from build123d import *

# Parameters (mm, degrees)
BOSS_EXTRUDE2_DEPTH     = 50.8
SKETCH2_R               = 12.7
CUT_EXTRUDE1_DEPTH      = 3.175
SKETCH3_R               = 6.35
CUT_EXTRUDE2_DEPTH      = 118.131253835
CUT_EXTRUDE3_DEPTH      = 117.397422652
CUT_EXTRUDE3_DEPTH_BACK = 117.397422652
SKETCH5_R               = 3.175
CUT_EXTRUDE4_DEPTH      = 118.946015193


with BuildPart() as part:
    # Sketch1 → Boss-Extrude2 (new body)
    with BuildSketch(Plane.XY):
        with BuildLine():
            Line((29.919216233, -6.35), (24.593444248, -6.35))
            ThreePointArc((24.593444248, -6.35), (23.905382985, -8.584443158), (23.014781645, -10.746154003))
            ThreePointArc((23.014781645, -10.746154003), (25.826619655, -7.542321317), (29.919216233, -6.35))
        make_face()
        with BuildLine():
            ThreePointArc((23.01478179, 10.746153692), (23.905383043, 8.584442996), (24.593444248, 6.35))
            Line((24.593444248, 6.35), (29.919216228, 6.35))
            ThreePointArc((29.919216228, 6.35), (25.826619797, 7.542321227), (23.01478179, 10.746153692))
        make_face()
        with BuildLine():
            Line((29.919216228, 6.35), (24.593444248, 6.35))
            ThreePointArc((24.593444248, 6.35), (25.197554285, 3.200509029), (25.4, 0))
            ThreePointArc((25.4, 0), (25.197554285, -3.200509029), (24.593444248, -6.35))
            Line((24.593444248, -6.35), (29.919216233, -6.35))
            Line((29.919216233, -6.35), (101.6, -6.35))
            Line((101.6, -6.35), (101.6, 6.35))
            Line((101.6, 6.35), (29.919216228, 6.35))
        make_face()
        with BuildLine():
            Line((24.593444248, -6.35), (0, -6.35))
            Line((0, -6.35), (0, -25.4))
            ThreePointArc((0, -25.4), (13.641988278, -21.425595811), (23.014781645, -10.746154003))
            ThreePointArc((23.014781645, -10.746154003), (23.905382985, -8.584443158), (24.593444248, -6.35))
        make_face()
        with BuildLine():
            Line((24.593444248, 6.35), (0, 6.35))
            Line((0, 6.35), (0, -6.35))
            Line((0, -6.35), (24.593444248, -6.35))
            ThreePointArc((24.593444248, -6.35), (25.197554285, -3.200509029), (25.4, 0))
            ThreePointArc((25.4, 0), (25.197554285, 3.200509029), (24.593444248, 6.35))
        make_face()
        with BuildLine():
            Line((0, 25.4), (0, 6.35))
            Line((0, 6.35), (24.593444248, 6.35))
            ThreePointArc((24.593444248, 6.35), (23.905383043, 8.584442996), (23.01478179, 10.746153692))
            ThreePointArc((23.01478179, 10.746153692), (13.641988422, 21.425595718), (0, 25.4))
        make_face()
        with BuildLine():
            Line((0, -6.35), (0, 6.35))
            Line((0, 6.35), (0, 25.4))
            ThreePointArc((0, 25.4), (-25.4, 0), (0, -25.4))
            Line((0, -25.4), (0, -6.35))
        make_face()
    extrude(amount=BOSS_EXTRUDE2_DEPTH)

    # Sketch2 → Cut-Extrude1 (cut)
    with BuildSketch(Plane(origin=(0, 6.35, 0), x_dir=(1, 0, 0), z_dir=(0, 1, 0))):
        with Locations(Location((76.2, -25.4, 0), (0, 0, 270))):
            Circle(SKETCH2_R)
    extrude(amount=-CUT_EXTRUDE1_DEPTH, mode=Mode.SUBTRACT)

    # Sketch3 → Cut-Extrude2 (cut, through all)
    with BuildSketch(Plane(origin=(0, 3.175, 0), x_dir=(1, 0, 0), z_dir=(0, 1, 0))):
        with Locations(Location((76.2, -25.4, 0), (0, 0, 270))):
            Circle(SKETCH3_R)
    extrude(amount=-CUT_EXTRUDE2_DEPTH, mode=Mode.SUBTRACT)

    # Sketch4 → Cut-Extrude3 (cut, two sides: drawn at the far end of the back side and taken through both)
    with BuildSketch(Plane.XY.offset(50.8).offset(-CUT_EXTRUDE3_DEPTH_BACK)):
        with BuildLine():
            Line((-12.296722124, 3.175), (-25.200781238, 3.175))
            ThreePointArc((-25.200781238, 3.175), (-25.350146385, 1.590621979), (-25.4, 0))
            ThreePointArc((-25.4, 0), (-25.350146385, -1.590621979), (-25.200781238, -3.175))
            Line((-25.200781238, -3.175), (-12.296722124, -3.175))
            ThreePointArc((-12.296722124, -3.175), (-12.7, 0), (-12.296722124, 3.175))
        make_face()
        with BuildLine():
            ThreePointArc((12.7, 0), (1.600254515, 12.598777143), (-12.296722124, 3.175))
            Line((-12.296722124, 3.175), (0, 3.175))
            Line((0, 3.175), (0, -3.175))
            Line((0, -3.175), (-12.296722124, -3.175))
            ThreePointArc((-12.296722124, -3.175), (1.600254515, -12.598777143), (12.7, 0))
        make_face()
        with BuildLine():
            Line((0, 3.175), (-12.296722124, 3.175))
            ThreePointArc((-12.296722124, 3.175), (-12.7, 0), (-12.296722124, -3.175))
            Line((-12.296722124, -3.175), (0, -3.175))
            Line((0, -3.175), (0, 3.175))
        make_face()
    extrude(amount=CUT_EXTRUDE3_DEPTH + CUT_EXTRUDE3_DEPTH_BACK, mode=Mode.SUBTRACT)

    # Sketch5 → Cut-Extrude4 (cut, through all)
    with BuildSketch(Plane(origin=(0, 6.35, 0), x_dir=(1, 0, 0), z_dir=(0, 1, 0))):
        with Locations(Location((44.45, -12.7, 0), (0, 0, 270))):
            Circle(SKETCH5_R)
        with Locations(Location((44.45, -38.1, 0), (0, 0, 270))):
            Circle(SKETCH5_R)
    extrude(amount=-CUT_EXTRUDE4_DEPTH, mode=Mode.SUBTRACT)


solid = part.part
Work out the finished part from the listing and answer in its coordinate system (mm). A direction names the side the tool comes from. Coordinates: 2 decimals unless noted, no trailing zeros. Write each loop counter-clockwise with the first axis right and the second up, starting at its lowest first coordinate (ties: lowest second). Pieces come first, ordered by that corner, then holes. Notation, with made-up numbers: M 76,33 L 134,33 A7 ccw 134,43 Z; hole C 52,81.5 d11. An arc over 180 degrees is marked long. Answer as CSV lines item,"result". Start each with the question number.
Item 1: Determine the mould class of faces 5 (the face through (46.596, 0.089, 35.76)), 6 (the face through (25.776, -7.575, 25.044)), 7 (the face through (-19, 3.175, 25)) for opening direction X: released by +X, released by -X, zero draft, split by the parting line, or undercut.
Item 2: A tool of negligible diameter and unlimited length cuts with its end or side. For faces 1 (the face through (63.8, 4.78, 22.65)), 2 (the face through (65, -6.35, 25)), 3 (the face through (58, 6.35, 25)), 4 (the face through (-19, -3.175, 25)), from which of +Z, -Z, +X, -X, +Y, -Y can it reach the whole face along a straight path? Write none if from no direction.
Item 3: Section C-C on x = 76.2 is taken. Write down the section's boundary in (y, z) (3 decimals), and give its area (3 significant figures).
Item 4: Flat-ended cylindrical pins translate along their axes: P1, Ø2, axis at y = 2, z = 21, coming from the -X side; P2, Ø4, axis at x = 63.5, z = 36, coming from the +Y side; P3, Ø4, axis at x = -16, z = 37, coming from the +Y side; P4, Ø5.5, axis at x = 44.45, z = 38.1, coming from the +Y side. Find the tip coordinate at first contact, or state that the pin passes through.
Item 5: Consider L1, parallel to X at y = 6, z = 27.5; L2, parallel to X at y = 4.7, z = 25.4; L3, parallel to Z at x = 47, y = -6. Determine where each line is inside the solid, lowest interval first.
Item 6: Section D-D on x = 93 is taken. Write down the section's boundary in (y, z).
Item 7: Section B-B on z = 25.4 is taken. Write down the section's boundary in (x, y) (3 decimals).
Item 8: Section A-A on x = 44.45 is taken. Write down the section's boundary in (y, z) (3 decimals).
Checks:
1,face 5,"undercut"
1,face 6,"released by +X"
1,face 7,"zero draft"
2,face 1,"+Y"
2,face 2,"+Z, -Z, +X, -Y"
2,face 3,"+Z, -Z, +X, +Y"
2,face 4,"+Z, -Z, -X"
3,outline,"M -6.35,0 L 6.35,0 L 6.35,12.7 L 3.175,12.7 L 3.175,19.05 L -6.35,19.05 Z; M -6.35,31.75 L 3.175,31.75 L 3.175,38.1 L 6.35,38.1 L 6.35,50.8 L -6.35,50.8 Z"
3,area,"444 mm²"
4,P1,"stops at x = 12.34"
4,P2,"stops at y = 6.35"
4,P3,"stops at y = 21.19"
4,P4,"passes through"
5,L1,"x = -24.68 to -11.19, 11.19 to 63.67, 88.73 to 101.6"
5,L2,"x = -24.96 to -11.8, 11.8 to 63.5, 88.9 to 101.6"
5,L3,"z = 0 to 10.81, 14.59 to 36.21, 39.99 to 50.8"
6,outline,"M -6.35,0 L 6.35,0 L 6.35,50.8 L -6.35,50.8 Z"
7,outline,"M -25.201,-3.175 A25.4 ccw 23.015,-10.746 A7.62 cw 29.919,-6.35 L 69.85,-6.35 L 69.85,3.175 L 63.5,3.175 L 63.5,6.35 L 29.919,6.35 A7.62 cw 23.015,10.746 A25.4 ccw -25.201,3.175 L -12.297,3.175 A12.7 cw long -12.297,-3.175 Z; M 82.55,-6.35 L 101.6,-6.35 L 101.6,6.35 L 88.9,6.35 L 88.9,3.175 L 82.55,3.175 Z"
8,outline,"M -6.35,0 L 6.35,0 L 6.35,9.525 L -6.35,9.525 Z; M -6.35,15.875 L 6.35,15.875 L 6.35,34.925 L -6.35,34.925 Z; M -6.35,41.275 L 6.35,41.275 L 6.35,50.8 L -6.35,50.8 Z"
